The model under review builds one solid part; all positions refer to its coordinate system, in mm. Coordinates: 2 decimals unless noted, no trailing zeros. Write each loop counter-clockwise with the first axis right and the second up, starting at its lowest first coordinate (ties: lowest second). Pieces come first, ordered by that corner, then holes.
Autodesk Inventor part; units mm, degrees
ref_plane "YZ Plane" through (0, 0, 0) normal (1, 0, 0) x (0, 1, 0)
ref_plane "XZ Plane" through (0, 0, 0) normal (0, 1, 0) x (-1, 0, 0)
ref_plane "XY Plane" through (0, 0, 0) normal (0, 0, 1) x (1, 0, 0)
sketch "Esboço1" plane through (0, 0, 0) normal (0, 1, 0) x (-1, 0, 0)
  line L0 (0, 0) -> (0, 150)
  line L1 (0, 150) -> (45, 150)
  line L2 (45, 150) -> (45, 0)
  line L3 (45, 0) -> (0, 0)
  line L4 (45, 0) -> (55, 0)
  circle A0 centre (5, 5) radius 2.5
  circle A1 centre (5, 145) radius 2.5
  circle A2 centre (40, 145) radius 2.5
  circle A3 centre (40, 5) radius 2.5
  circle A4 centre (40.2, 112.5) radius 2.5
  circle A5 centre (4.8, 112.5) radius 2.5
  circle A6 centre (40.2, 37.5) radius 2.5
  circle A7 centre (4.8, 37.5) radius 2.5
  dimension "d0" = 150
  dimension "d1" = 45
  dimension "d10" = 5
  dimension "d12" = 5
  dimension "d22" = 5
  dimension "d23" = 5
  dimension "d35" = 5
  dimension "d36" = 5
  dimension "d37" = 5
  dimension "d38" = 5
extrude "Extrusão6" add sketch "Esboço1" along normal blind 5
properties part number "BaseM"
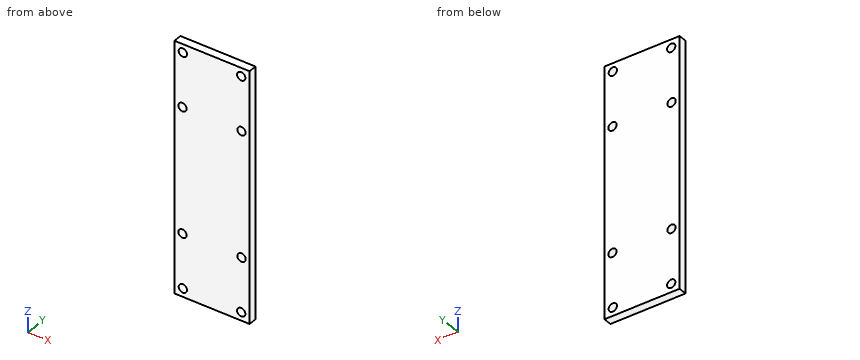
Item 1: To check wall thickness, follow line 1 along Z through (x, y) = (-40, 1.75); line 2 along X through (y, z) = (1.2, 145); line 3 along Z through (x, y) = (-3, 0.85). State the ranges of each line that lie inside material, in increasing order.
Solved:
line 1: z = 0 to 2.5, 7.5 to 35.01, 39.99 to 110.01, 114.99 to 142.5, 147.5 to 150
line 2: x = -45 to -42.5, -37.5 to -7.5, -2.5 to 0
line 3: z = 0 to 3.5, 6.5 to 35.77, 39.23 to 110.77, 114.23 to 143.5, 146.5 to 150
Item 2: Take a section at A-A, the plane y = 3.8. Count the separate pieces of the cut face and the enclosed holes in it, plus the area to 3 significant figures.
Solved:
separate pieces: 1
enclosed holes: 8
area: 6,590 mm2
Item 3: For pin 1 (12 mm diameter, centred on x = -26.5, z = 86, fed in from -Y), flat-tipped, find the tip position at first contact; note if it passes through.
Solved:
pin 1: stops at y = 0
Item 4: Take a section at B-B, the plane z = 112.5. Write out the cut boundary in (x, y), plus the area to 3 significant figures.
Solved:
outline: (-45, 0) - (-42.7, 0) - (-42.7, 5) - (-45, 5) - close; (-37.7, 0) - (-7.3, 0) - (-7.3, 5) - (-37.7, 5) - close; (-2.3, 0) - (0, 0) - (0, 5) - (-2.3, 5) - close
area: 175 mm2
Item 5: Take a section at C-C, the plane x = -40. Write out the cut boundary in (y, z), plus the area to 3 significant figures.
Solved:
outline: (0, 0) - (5, 0) - (5, 2.5) - (0, 2.5) - close; (0, 7.5) - (5, 7.5) - (5, 35.01) - (0, 35.01) - close; (0, 39.99) - (5, 39.99) - (5, 110.01) - (0, 110.01) - close; (0, 114.99) - (5, 114.99) - (5, 142.5) - (0, 142.5) - close; (0, 147.5) - (5, 147.5) - (5, 150) - (0, 150) - close
area: 650 mm2
